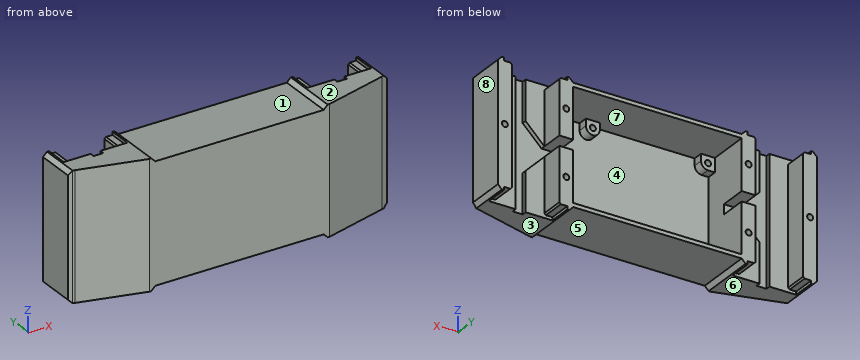
```python
from build123d import *

# Parameters (mm, degrees)
SKETCH2_W            = 85
SKETCH2_H            = 56
BOSS_EXTRUDE4_DEPTH  = 3
SKETCH3_W            = 89
SKETCH3_H            = 60
SKETCH3_W_2          = 85
SKETCH3_H_2          = 56
BOSS_EXTRUDE5_DEPTH  = 29
SKETCH5_R            = 3.5
BOSS_EXTRUDE10_DEPTH = 8
CUT_EXTRUDE1_DEPTH   = 11.7
CHAMFER1_SIZE        = 2
CUT_EXTRUDE2_DEPTH   = 11.7
SKETCH8_W            = 64
SKETCH8_H            = 29
BOSS_EXTRUDE11_DEPTH = 2
SKETCH9_W            = 64
SKETCH9_H            = 29
BOSS_EXTRUDE12_DEPTH = 2
CHAMFER2_SIZE        = 2
CHAMFER3_SIZE        = 0.75
CUT_EXTRUDE4_DEPTH   = 107.851532511
SKETCH10_W           = 7.0025
SKETCH10_H           = 5
SKETCH10_W_2         = 85
SKETCH10_W_3         = 7
CUT_EXTRUDE5_DEPTH   = 14
CHAMFER4_SIZE        = 9.5
SKETCH14_R           = 1.5
CUT_EXTRUDE7_DEPTH   = 5
SKETCH15_R           = 1.5
CUT_EXTRUDE8_DEPTH   = 5


with BuildPart() as part:
    # Sketch2 → Boss-Extrude4 (new body)
    with BuildSketch(Plane(origin=(0, 0, 0), x_dir=(1, 0, 0), z_dir=(0, 1, 0))):
        Rectangle(SKETCH2_W, SKETCH2_H)
    extrude(amount=BOSS_EXTRUDE4_DEPTH)

    # Sketch3 → Boss-Extrude5 (add)
    # profile 1 of 3: a face of its own
    with BuildSketch(Plane(origin=(0, 0, 0), x_dir=(1, 0, 0), z_dir=(0, 1, 0))):
        Rectangle(SKETCH3_W, SKETCH3_H)
        Rectangle(SKETCH3_W_2, SKETCH3_H_2, mode=Mode.SUBTRACT)
    # profile 2 of 3: a face of its own
    with BuildSketch(Plane(origin=(0, 0, 0), x_dir=(1, 0, 0), z_dir=(0, 1, 0))):
        Polygon((-78.5, -32), (-44.5, -32), (-44.5, -30), (-44.5, 30), (-44.5, 32), (-78.5, 32), (-78.5, 0), align=None)
    # profile 3 of 3: a face of its own
    with BuildSketch(Plane(origin=(0, 0, 0), x_dir=(1, 0, 0), z_dir=(0, 1, 0))):
        Polygon((44.5, -32), (44.5, -30), (44.5, 30), (44.5, 32), (78.5, 32), (78.5, 0), (78.5, -32), align=None)
    extrude(amount=BOSS_EXTRUDE5_DEPTH)

    # Sketch5 → Boss-Extrude10 (add)
    with BuildSketch(Plane(origin=(0, 0, 0), x_dir=(1, 0, 0), z_dir=(0, 1, 0))):
        with Locations((-39, 24.5)):
            Circle(SKETCH5_R)
        with BuildLine():
            ThreePointArc((-42.5, 24.5), (-41.474873734, 26.974873734), (-39, 28))
            Line((-39, 28), (-42.5, 28))
            Line((-42.5, 28), (-42.5, 24.5))
        make_face()
        with BuildLine():
            ThreePointArc((-39, 21), (-41.474873734, 22.025126266), (-42.5, 24.5))
            Line((-42.5, 24.5), (-42.5, 21))
            Line((-42.5, 21), (-39, 21))
        make_face()
        with BuildLine():
            Line((-35.5, 24.5), (-35.5, 28))
            Line((-35.5, 28), (-39, 28))
            ThreePointArc((-39, 28), (-36.525126266, 26.974873734), (-35.5, 24.5))
        make_face()
        with BuildLine():
            ThreePointArc((-35.5, -24.5), (-36.525126266, -26.974873734), (-39, -28))
            Line((-39, -28), (-35.5, -28))
            Line((-35.5, -28), (-35.5, -24.5))
        make_face()
        with Locations((-39, -24.5)):
            Circle(SKETCH5_R)
        with BuildLine():
            ThreePointArc((-39, -28), (-41.474873734, -26.974873734), (-42.5, -24.5))
            Line((-42.5, -24.5), (-42.5, -28))
            Line((-42.5, -28), (-39, -28))
        make_face()
        with BuildLine():
            Line((-39, -21), (-42.5, -21))
            Line((-42.5, -21), (-42.5, -24.5))
            ThreePointArc((-42.5, -24.5), (-41.474873734, -22.025126266), (-39, -21))
        make_face()
        with BuildLine():
            Line((19.08999999, -28), (22.59, -28))
            Line((22.59, -28), (22.59, -24.5))
            ThreePointArc((22.59, -24.5), (21.564873731, -26.974873738), (19.08999999, -28))
        make_face()
        with Locations((19.09, -24.5)):
            Circle(SKETCH5_R)
        with BuildLine():
            Line((15.59, -28), (19.08999999, -28))
            ThreePointArc((19.08999999, -28), (16.615126262, -26.974873731), (15.59, -24.5))
            Line((15.59, -24.5), (15.59, -28))
        make_face()
        with BuildLine():
            ThreePointArc((19.09, 28), (21.564873734, 26.974873734), (22.59, 24.5))
            Line((22.59, 24.5), (22.59, 28))
            Line((22.59, 28), (19.09, 28))
        make_face()
        with BuildLine():
            Line((15.59, 28), (15.59, 24.5))
            ThreePointArc((15.59, 24.5), (16.615126266, 26.974873734), (19.09, 28))
            Line((19.09, 28), (15.59, 28))
        make_face()
        with Locations((19.09, 24.5)):
            Circle(SKETCH5_R)
    extrude(amount=BOSS_EXTRUDE10_DEPTH)

    # Sketch6 → Cut-Extrude1 (cut)
    with BuildSketch(Plane(origin=(0, 29, 0), x_dir=(1, 0, 0), z_dir=(0, 1, 0))):
        Polygon((-73.5025, 30.43), (-49.5025, 30.43), (-45.48, 30.43), (-45.48, 32), (-77.53, 32), (-77.53, 30.43), align=None)
        Polygon((-73.5025, -30.43), (-49.5025, -30.43), (-49.5025, 0), (-49.5025, 30.43), (-73.5025, 30.43), (-73.5025, 0), align=None)
        Polygon((-77.525, -32), (-45.475, -32), (-45.475, -30.43), (-49.5025, -30.43), (-73.5025, -30.43), (-77.525, -30.43), align=None)
    extrude(amount=-CUT_EXTRUDE1_DEPTH, mode=Mode.SUBTRACT)

    # Chamfer1
    chamfer1_edges = [part.edges().sort_by_distance(p)[0] for p in [
        (-44.5, 14.5, 30),
        (44.5, 14.5, 30),
        (44.5, 14.5, -30),
        (-44.5, 14.5, -30),
    ]]
    chamfer(chamfer1_edges, length=CHAMFER1_SIZE - 0.0001)  # a hair under: the kernel refuses the full size

    # Sketch7 → Cut-Extrude2 (cut)
    with BuildSketch(Plane(origin=(0, 29, 0), x_dir=(1, 0, 0), z_dir=(0, 1, 0))):
        Polygon((61.5, 32), (45.475, 32), (45.475, 30.43), (49.5, 30.43), (49.5, -30.43), (45.47, -30.43), (45.47, -32), (61.5, -32), (77.53, -32), (77.53, -30.43), (73.5, -30.43), (73.5, 30.43), (77.53, 30.43), (77.53, 32), align=None)
    extrude(amount=-CUT_EXTRUDE2_DEPTH, mode=Mode.SUBTRACT)

    # Sketch8 → Boss-Extrude11 (add)
    with BuildSketch(Plane.ZY.offset(78.5)):
        with Locations((0, 14.5)):
            Rectangle(SKETCH8_W, SKETCH8_H)
    extrude(amount=BOSS_EXTRUDE11_DEPTH)

    # Sketch9 → Boss-Extrude12 (add)
    with BuildSketch(Plane(origin=(78.5, 0, 0), x_dir=(0, 0, -1), z_dir=(1, 0, 0))):
        with Locations((0, 14.5)):
            Rectangle(SKETCH9_W, SKETCH9_H)
    extrude(amount=BOSS_EXTRUDE12_DEPTH)

    # Chamfer2
    chamfer2_edges = [part.edges().sort_by_distance(p)[0] for p in [
        (-80.5, 14.5, -32),
        (-80.5, 14.5, 32),
        (80.5, 14.5, 32),
        (80.5, 14.5, -32),
    ]]
    chamfer(chamfer2_edges, length=CHAMFER2_SIZE)

    # Chamfer3
    chamfer3_edges = [part.edges().sort_by_distance(p)[0] for p in [
        (-73.5025, 23.15, -30.43),
        (-49.5025, 23.15, -30.43),
        (-49.5025, 23.15, 30.43),
        (-73.5025, 23.15, 30.43),
        (73.5, 23.15, -30.43),
        (73.5, 23.15, 30.43),
        (49.5, 23.15, 30.43),
        (49.5, 23.15, -30.43),
    ]]
    chamfer(chamfer3_edges, length=CHAMFER3_SIZE)

    # Sketch11 → Cut-Extrude4 (cut, through all)
    with BuildSketch(Plane.XY.offset(32)):
        Polygon((104.627072185, -13.366120131), (45.47, 0), (77.53, 8.65), (97.251349741, 13.97095057), align=None)
        Polygon((-80.747190975, -16.87538219), (-45.475, 0), (-78.5, 0), (-78.5, 8.913143526), (-93.850671493, 13.056148468), align=None)
        Polygon((-45.475, 0), (-77.525, 8.65), (-78.5, 8.913143526), (-78.5, 0), align=None)
    extrude(amount=-CUT_EXTRUDE4_DEPTH, mode=Mode.SUBTRACT)

    # Sketch10 → Cut-Extrude5 (cut)
    with BuildSketch(Plane(origin=(0, 29, 0), x_dir=(1, 0, 0), z_dir=(0, 1, 0))):
        Polygon((-59.005, -32), (-59.005, 32), (-61.505, 32), (-64.005, 32), (-64.005, -32), (-61.5, -32), align=None)
        Polygon((-49.5025, 2.5), (-59.005, 2.5), (-59.005, 0), (-59.005, -2.5), (-49.5025, -2.5), align=None)
        with Locations((-46.00125, 0)):
            Rectangle(SKETCH10_W, SKETCH10_H)
        Rectangle(SKETCH10_W_2, SKETCH10_H)
        with Locations((46, 0)):
            Rectangle(SKETCH10_W_3, SKETCH10_H)
        Polygon((59.0025, 2.5), (49.5, 2.5), (49.5, -2.5), (59.0025, -2.5), (59.0025, 0), align=None)
        Polygon((64.0025, -32), (64.0025, 32), (61.5025, 32), (59.0025, 32), (59.0025, -32), (61.5, -32), align=None)
    extrude(amount=-CUT_EXTRUDE5_DEPTH, mode=Mode.SUBTRACT)

    # Chamfer4
    chamfer4_edges = [part.edges().sort_by_distance(p)[0] for p in [
        (-59.005, 16.15, -2.5),
        (59.0025, 16.15, -2.5),
        (59.0025, 16.15, 2.5),
        (-59.005, 16.15, 2.5),
    ]]
    chamfer(chamfer4_edges, length=CHAMFER4_SIZE)

    # Sketch14 → Cut-Extrude7 (cut)
    with BuildSketch(Plane(origin=(0, 8, 0), x_dir=(1, 0, 0), z_dir=(0, 1, 0))):
        with Locations(Location((19.09, -24.5, 0), (0, 0, 270))):
            Circle(SKETCH14_R)
        with Locations(Location((-39, -24.5, 0), (0, 0, 270))):
            Circle(SKETCH14_R)
        with Locations(Location((-39, 24.5, 0), (0, 0, 270))):
            Circle(SKETCH14_R)
        with Locations(Location((19.09, 24.5, 0), (0, 0, 270))):
            Circle(SKETCH14_R)
    extrude(amount=-CUT_EXTRUDE7_DEPTH, mode=Mode.SUBTRACT)

    # Sketch15 → Cut-Extrude8 (cut)
    with BuildSketch(Plane(origin=(0, 29, 0), x_dir=(1, 0, 0), z_dir=(0, 1, 0))):
        with Locations(Location((46, 16.465, 0), (0, 0, 270))):
            Circle(SKETCH15_R)
        with Locations(Location((46, -16.465, 0), (0, 0, 270))):
            Circle(SKETCH15_R)
        with Locations(Location((77, 0, 0), (0, 0, 270))):
            Circle(SKETCH15_R)
        with Locations(Location((-46.0025, 16.465, 0), (0, 0, 270))):
            Circle(SKETCH15_R)
        with Locations(Location((-46.00125, -16.465, 0), (0, 0, 270))):
            Circle(SKETCH15_R)
        with Locations(Location((-77.00125, 0, 0), (0, 0, 270))):
            Circle(SKETCH15_R)
    extrude(amount=-CUT_EXTRUDE8_DEPTH, mode=Mode.SUBTRACT)


solid = part.part
```
Input: part model. Units: mm. Frame: model coordinates. Face numbers are marked on the shaded views. A direction names the side the tool comes from. Coordinates: 2 decimals unless noted, no trailing zeros. Write each loop counter-clockwise with the first axis right and the second up, starting at its lowest first coordinate (ties: lowest second). Pieces come first, ordered by that corner, then holes.
1) Material intervals for line 1 along X through (y, z) = (23.5, -20); line 2 along Z through (x, y) = (-13, 5); line 3 along Z through (x, y) = (77, 25.25), sorted ascending.
2) Set-up query: the marked faces 1, 2, 3, 4 and 5. Return all of +Z, -Z, +X, -X, +Y, -Y with unobstructed straight access to the full face (end or side cutting, diameter ignored); none if empty.
3) Section B-B on x = 8. Output: boundary loops of the cut face in (y, z), and give its area (3 significant figures).
4) Pin query (flat end, axial travel): pin 1 Ø2 at (x, y) = (-41, 9.5) entering from +Z; pin 2 Ø6 at (x, z) = (-30.5, 6.5) entering from +Y; pin 3 Ø5 at (x, z) = (59.5, -16.5) entering from +Y. Return the tip coordinate at first contact, or that it passes through.
5) Section D-D on y = 5.5. State how many separate pieces and enclosed holes the cut face has, and give its area (3 significant figures).
6) Mould query, pull axis Z, two halves, no side actions, for the marked faces 6, 7 and 8. Classes: pulls with the +Z half, pulls with the -Z half, needs draft (parallel to the pull), parting line crosses it, or undercut.
Check result:
1. line 1: x = -80.5 to -73.5, -49.5 to -42.5, 42.5 to 49.5, 73.5 to 80.5
1. line 2: z = -30 to -28, 28 to 30
1. line 3: z = -30.43 to -1.5, 1.5 to 30.43
2. face 1: +Z, +Y, -Y
2. face 2: +Z, +X, -X, +Y, -Y
2. face 3: -Z, +X, -X, +Y, -Y
2. face 4: +Y
2. face 5: -Z, +Y, -Y
3. outline: (0, -30) - (29, -30) - (29, -28) - (3, -28) - (3, 28) - (29, 28) - (29, 30) - (0, 30) - close
3. area: 284 mm2
4. pin 1: stops at z = 30
4. pin 2: stops at y = 3
4. pin 3: stops at y = 17.3
5. separate pieces: 1
5. enclosed holes: 5
5. area: 3,470 mm2
6. face 6: pulls with the -Z half
6. face 7: undercut
6. face 8: needs draft
